from build123d import *

# Parameters (mm, degrees)
F0_W     = 47.5
F0_H     = 43
F1_DEPTH = 0.9
F2_W     = 43.5
F2_H     = 39
F3_DEPTH = 1
F4_W     = 45.5
F4_H     = 42
F5_DEPTH = 0.3


with BuildPart() as f1:
    # F0 (on Front) → F1 (new body, symmetric)
    with BuildSketch(Plane.XZ):
        with Locations((23.75, 21.5)):
            Rectangle(F0_W, F0_H)
    extrude(amount=F1_DEPTH, both=True)

    # F2 (on Front) → F3 (cut, symmetric)
    with BuildSketch(Plane.XZ):
        with Locations((23.75, 21.5)):
            Rectangle(F2_W, F2_H)
    extrude(amount=F3_DEPTH, both=True, mode=Mode.SUBTRACT)

    # F4 (on Front) → F5 (cut, symmetric)
    with BuildSketch(Plane.XZ):
        with Locations((23.75, 22)):
            Rectangle(F4_W, F4_H)
    extrude(amount=F5_DEPTH, both=True, mode=Mode.SUBTRACT)


solid = f1.part
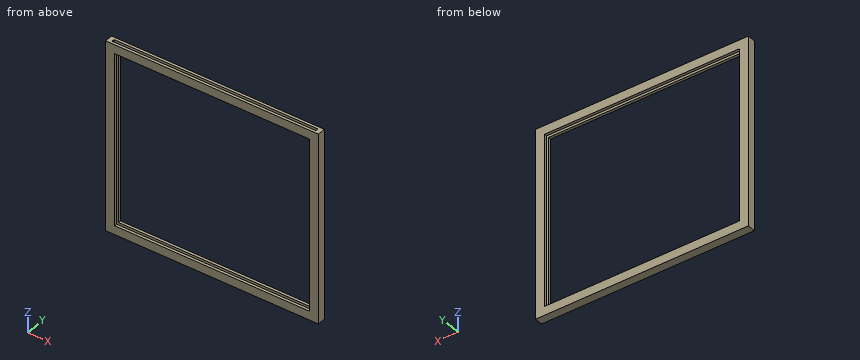
Can you work these out from the model? Positions are in its coordinate system, mm. Coordinates: 2 decimals unless noted, no trailing zeros. Write each loop counter-clockwise with the first axis right and the second up, starting at its lowest first coordinate (ties: lowest second). Pieces come first, ordered by that corner, then holes. Notation, with made-up numbers: (-8, 69.5) -> (42, 69.5) arc R18 cw to (42, 81.5) -> close; hole circle Ø7 at (44.25, 51). An arc over 180 degrees is marked (long way). Write each question's results on one line, items separated by ' | '. Start each with the question number.
Q1. Imagine slicing it at A-A (x = 29.5). Write out the boundary of the cut face in (y, z), then the cut area to 3 significant figures.
Q2. If I drill on probe 1 along Y at (x, z) = (46, 11.5); probe 2 along X at (y, z) = (-0.8, 10.5); probe 3 along Z at (x, y) = (18, 0.7), over which ranges is the centre line in solid material (lowest first)?
Q3. Imagine slicing it at B-B (z = 5.5). Write out the boundary of the cut face in (x, y), then the cut area to 3 significant figures.
Taken from the geometry:
1) outline: (-0.9, 0) -> (0.9, 0) -> (0.9, 2) -> (0.3, 2) -> (0.3, 1) -> (-0.3, 1) -> (-0.3, 2) -> (-0.9, 2) -> close; (-0.9, 41) -> (-0.3, 41) -> (-0.3, 43) -> (-0.9, 43) -> close; (0.3, 41) -> (0.9, 41) -> (0.9, 43) -> (0.3, 43) -> close | area: 5.40 mm^2
2) probe 1: y = -0.9 to -0.3, 0.3 to 0.9 | probe 2: x = 0 to 2, 45.5 to 47.5 | probe 3: z = 0 to 2, 41 to 43
3) outline: (0, -0.9) -> (2, -0.9) -> (2, -0.3) -> (1, -0.3) -> (1, 0.3) -> (2, 0.3) -> (2, 0.9) -> (0, 0.9) -> close; (45.5, -0.9) -> (47.5, -0.9) -> (47.5, 0.9) -> (45.5, 0.9) -> (45.5, 0.3) -> (46.5, 0.3) -> (46.5, -0.3) -> (45.5, -0.3) -> close | area: 6.00 mm^2
